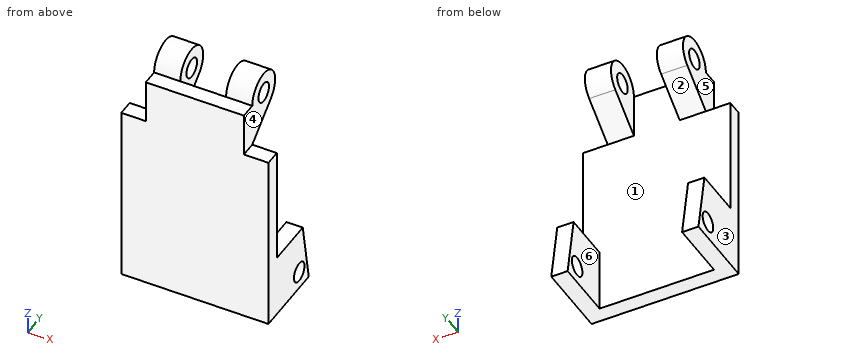
```python
from build123d import *

# Parameters (mm, degrees)
SKETCH1_W           = 57.15
SKETCH1_H           = 71.12
SKETCH1_W_2         = 38.1
SKETCH1_H_2         = 17.145
BOSS_EXTRUDE1_DEPTH = 6.0325
SKETCH2_R           = 8.255
SKETCH2_R_2         = 3.81
BOSS_EXTRUDE2_DEPTH = 38.1
SKETCH3_W           = 17.78
SKETCH3_H           = 25.4
CUT_EXTRUDE1_DEPTH  = 35.7505
SKETCH4_R           = 3.81
BOSS_EXTRUDE3_DEPTH = 57.15
SKETCH5_W           = 44.45
SKETCH5_H           = 23.0505
CUT_EXTRUDE2_DEPTH  = 35.7505


with BuildPart() as part:
    # Sketch1 → Boss-Extrude1 (new body)
    with BuildSketch(Plane(origin=(0, 0, 0), x_dir=(1, 0, 0), z_dir=(0, 1, 0))):
        with Locations((28.575, 35.56)):
            Rectangle(SKETCH1_W, SKETCH1_H)
        with Locations((28.575, -8.5725)):
            Rectangle(SKETCH1_W_2, SKETCH1_H_2)
    extrude(amount=BOSS_EXTRUDE1_DEPTH)

    # Sketch2 → Boss-Extrude2 (add)
    with BuildSketch(Plane.ZY.offset(-9.525)):
        with BuildLine():
            Line((10.691759465, 19.435384187), (0, 6.0325))
            Line((0, 6.0325), (17.145, 6.0325))
            ThreePointArc((17.145, 6.0325), (9.707231216, 10.706352067), (10.691759465, 19.435384187))
        make_face()
        with Locations((17.145, 14.2875)):
            Circle(SKETCH2_R)
        with Locations((17.145, 14.2875)):
            Circle(SKETCH2_R_2, mode=Mode.SUBTRACT)
    extrude(amount=-BOSS_EXTRUDE2_DEPTH)

    # Sketch3 → Cut-Extrude1 (cut)
    with BuildSketch(Plane(origin=(0, 6.0325, 0), x_dir=(1, 0, 0), z_dir=(0, 1, 0))):
        with Locations((28.575, -12.7)):
            Rectangle(SKETCH3_W, SKETCH3_H)
    extrude(amount=CUT_EXTRUDE1_DEPTH, mode=Mode.SUBTRACT)

    # Sketch4 → Boss-Extrude3 (add)
    with BuildSketch(Plane.ZY):
        Polygon((-46.355, 6.0325), (-46.355, 24.765), (-71.12, 29.083), (-71.12, 6.0325), align=None)
        with Locations((-64.135, 22.225)):
            Circle(SKETCH4_R, mode=Mode.SUBTRACT)
    extrude(amount=-BOSS_EXTRUDE3_DEPTH)

    # Sketch5 → Cut-Extrude2 (cut)
    with BuildSketch(Plane(origin=(0, 0, -71.12), x_dir=(-1, 0, 0), z_dir=(0, 0, -1))):
        with Locations((-28.575, 17.55775)):
            Rectangle(SKETCH5_W, SKETCH5_H)
    extrude(amount=-CUT_EXTRUDE2_DEPTH, mode=Mode.SUBTRACT)


solid = part.part
```
The listing builds one solid part. Answer for the finished solid, in the listing's coordinates (mm). Face numbers are marked on the shaded views. A direction names the side the tool comes from. Give positions to 0.01 mm unless a question says otherwise; leave off trailing zeros. Order: outer loops, then holes, each group sorted by start corner. A loop starts at its lowest first (then second) coordinate and runs counter-clockwise, first axis right, second up. Notation, with made-up numbers: (46.5, 86.25) -> (99.5, 86.25) arc R23 cw to (99.5, 94.25) -> close; hole circle Ø7 at (-24.5, -13.5). An arc over 180 degrees is marked (long way). Answer as a JSON object with one key per item and string values. Group by question number.
Item 1: Flat-ended cylindrical pins translate along their axes: pin 1 (12 mm diameter, centred on y = 14.29, z = 17.14, fed in from -X) (3 decimals); pin 2 (2 mm diameter, centred on x = 9, y = 8, fed in from +Z); pin 3 (8 mm diameter, centred on x = 28, z = -43.5, fed in from +Y). Find the tip coordinate at first contact, or state that the pin passes through.
Item 2: The part is cut by section C-C on z = -19.5. Write down the section's boundary in (x, y).
Item 3: The part is cut by section D-D on x = 22.5. Write down the section's boundary in (y, z) (1 decimal), and give its area (3 significant figures).
Item 4: A tool of negligible diameter and unlimited length cuts with its end or side. For the marked faces 4, 5 and 6, from which of +Z, -Z, +X, -X, +Y, -Y can it reach the whole face along a straight path? Write none if from no direction.
Item 5: The part is cut by section B-B on z = -63.5. Write down the section's boundary in (x, y), and give its area (3 significant figures).
Item 6: The part is cut by section A-A on x = 38.5. Write down the section's boundary in (y, z) (1 decimal).
Item 7: Consider L1, parallel to X at y = 17.5, z = 14 (3 decimals); L2, parallel to X at y = 8.5, z = -51.5; L3, parallel to X at y = 4.75, z = 13 (3 decimals). Determine where each line is inside the solid, lowest interval first. Write a range as from..to.
Item 8: Determine the mould class of the marked faces 1, 2 and 3 for opening direction X: pulls with the +X half, pulls with the -X half, needs draft (parallel to the pull), parting line crosses it, or undercut.
Result set:
{
 "1": {"pin 1": "x = 9.525", "pin 2": "z = 23.36", "pin 3": "y = 6.03"},
 "2": {"outline": "(0, 0) -> (57.15, 0) -> (57.15, 6.03) -> (0, 6.03) -> close"},
 "3": {"outline": "(0, -71.1) -> (6, -71.1) -> (6, 17.1) -> (0, 17.1) -> close", "area": "532 mm²"},
 "4": {"face 4": "+Z, +X, +Y, -Y", "face 5": "+Z, -X, +Y, -Y", "face 6": "+Z, -Z, +Y"},
 "5": {"outline": "(0, 0) -> (57.15, 0) -> (57.15, 18.47) -> (50.8, 18.47) -> (50.8, 6.03) -> (6.35, 6.03) -> (6.35, 18.47) -> (0, 18.47) -> close; (0, 25.98) -> (6.35, 25.98) -> (6.35, 27.75) -> (0, 27.75) -> close; (50.8, 25.98) -> (57.15, 25.98) -> (57.15, 27.75) -> (50.8, 27.75) -> close", "area": "525 mm²"},
 "6": {"outline": "(0, -71.1) -> (6, -71.1) -> (6, 0) -> (19.4, 10.7) arc R8.3 ccw (long way) to (6, 17.1) -> (0, 17.1) -> close; hole circle Ø7.6 at (14.3, 17.1)"},
 "7": {"L1": "9.525..19.685, 37.465..47.625", "L2": "0..6.35, 50.8..57.15", "L3": "9.525..47.625"},
 "8": {"face 1": "undercut", "face 2": "needs draft", "face 3": "pulls with the -X half"}
}
